```python
from build123d import *

# Parameters (mm, degrees)
BOSS_EXTRUDE1_DEPTH = 30
FILLET1_R           = 20
SKETCH2_R           = 6
CUT_EXTRUDE1_DEPTH  = 97.2


with BuildPart() as part:
    # Sketch1 → Boss-Extrude1 (new body)
    with BuildSketch(Plane(origin=(0, 0, 0), x_dir=(1, 0, 0), z_dir=(0, 1, 0))):
        Polygon((0, 115), (-10, 115), (-10, -10), (86.2, -10), (86.2, 115), (76.2, 115), (76.2, 0), (0, 0), align=None)
    extrude(amount=BOSS_EXTRUDE1_DEPTH)

    # Fillet1
    fillet1_edges = [part.edges().sort_by_distance(p)[0] for p in [
        (86.2, 15, 10),
        (-10, 15, 10),
    ]]
    fillet(fillet1_edges, radius=FILLET1_R)

    # Sketch2 → Cut-Extrude1 (cut, through all)
    with BuildSketch(Plane(origin=(86.2, 0, 0), x_dir=(0, 0, -1), z_dir=(1, 0, 0))):
        with Locations((100, 15)):
            Circle(SKETCH2_R)
    extrude(amount=-CUT_EXTRUDE1_DEPTH, mode=Mode.SUBTRACT)


solid = part.part
```
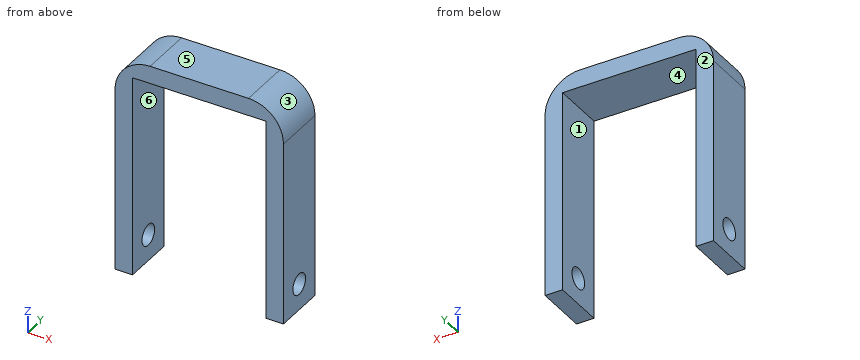
Source: CAD feature listing. Evaluate the final solid. Frame: model axes, mm. Face numbers are marked on the shaded views. A direction names the side the tool comes from. Coordinates: 2 decimals unless noted, no trailing zeros. Order: outer loops, then holes, each group sorted by start corner. A loop starts at its lowest first (then second) coordinate and runs counter-clockwise, first axis right, second up. Notation, with made-up numbers: M -39.75,68 L -6.75,68 A21 cw -6.75,80 Z; hole C 14.5,2.5 d9. An arc over 180 degrees is marked long. Write each question's results on one line, items separated by ' | '. Start each with the question number.
1) Access query for the marked faces 1 and 2. Directions: +Z, -Z, +X, -X, +Y, -Y. A direction counts if a zero-diameter tool reaches every point of the face in a straight line with its end or side. Return the directions, or none.
2) Line query: line 1 (Y direction, x = 81, z = -100); line 2 (X direction, y = 21, z = -42.5); line 3 (Z direction, x = 14, y = 9.5). Output: solid intervals per line, ascending. Write a range as from..to.
3) Contact query for flat-ended pins moving along their axis: pin 1 Ø8 at (x, y) = (7.5, 21) entering from -Z; pin 2 Ø5 at (y, z) = (10, -5.5) entering from -X. Output: stop coordinate, or through.
4) Section query D-D (z = -57.5). Return the cut outline in (x, y), plus the area to 3 significant figures.
5) Section query C-C (y = 25.25). Return the cut outline in (x, z), plus the area to 3 significant figures.
6) Section query A-A (y = 15). Return the cut outline in (x, z).
7) Draft query along X for the marked faces 3, 4, 5 and 6. Return one class per face: released by +X, released by -X, zero draft, split by the parting line, or undercut.
8) Section query B-B (z = -100). Return the cut outline in (x, y).
Answers:
1) face 1: -Z, +Y, -Y | face 2: +Z, -Z, +X, -X, +Y
2) line 1: y = 0..9, 21..30 | line 2: x = -10..0, 76.2..86.2 | line 3: z = 0..10
3) pin 1: stops at z = 0 | pin 2: stops at x = -9.9
4) outline: M -10,0 L 0,0 L 0,30 L -10,30 Z; M 76.2,0 L 86.2,0 L 86.2,30 L 76.2,30 Z | area: 600 mm^2
5) outline: M -10,-115 L 0,-115 L 0,0 L 76.2,0 L 76.2,-115 L 86.2,-115 L 86.2,-10 A20 ccw 66.2,10 L 10,10 A20 ccw -10,-10 Z | area: 3,090 mm^2
6) outline: M -10,-115 L 0,-115 L 0,-106 L -10,-106 Z; M -10,-94 L 0,-94 L 0,0 L 76.2,0 L 76.2,-94 L 86.2,-94 L 86.2,-10 A20 ccw 66.2,10 L 10,10 A20 ccw -10,-10 Z; M 76.2,-115 L 86.2,-115 L 86.2,-106 L 76.2,-106 Z
7) face 3: released by +X | face 4: undercut | face 5: zero draft | face 6: undercut
8) outline: M -10,0 L 0,0 L 0,9 L -10,9 Z; M -10,21 L 0,21 L 0,30 L -10,30 Z; M 76.2,0 L 86.2,0 L 86.2,9 L 76.2,9 Z; M 76.2,21 L 86.2,21 L 86.2,30 L 76.2,30 Z
